The figure shows three views and two pictorial views of one solid part (mm, origin at its lowest corner). Answer the questions. A direction names the side the tool comes from. Coordinates: 2 decimals unless noted, no trailing zeros. Order: outer loops, then holes, each group sorted by start corner. A loop starts at its lowest first (then second) coordinate and runs counter-clockwise, first axis right, second up. Notation, with made-up numbers: M -35.5,74.5 L -4.5,74.5 A31 cw -4.5,109.5 Z; hole C -21,78 d3. An arc over 180 degrees is marked long. Answer in a Markdown table with one row per item. Add a question column.
Item 1: The part is cut by section C-C (y = 11.25). Write down the section's boundary in (x, z).
Item 2: Flat-ended cylindrical pins translate along their axes: pin 1 Ø7.5 at (x, y) = (31, 4.5) entering from -Z; pin 2 Ø4.5 at (y, z) = (6, 13.5) entering from +X. Find the tip coordinate at first contact, or state that the pin passes through.
Item 3: The part is cut by section A-A (x = 4.75). Write down the section's boundary in (y, z).
Item 4: Consider line 1 (Z direction, x = 4.75, y = 7.5); line 2 (Z direction, x = 47.75, y = 10); line 3 (Z direction, x = 22, y = 11.5). Determine where each line is inside the solid, lowest interval first. Write a range as from..to.
Item 5: Which of the six approach directions +Z, -Z, +X, -X, +Y, -Y give full straight-line access (tool end or side, diameter ignored) to the marked faces 1 and 2?
Item 6: The part is cut by section B-B (z = 44.75). Write down the section's boundary in (x, y).
Item 7: The mould has two halves that part along Z. Classify the marked faces 3, 4, 5 and 6: released by +Z, released by -Z, zero draft, split by the parting line, or undercut.
Item 8: The part is cut by section D-D (x = 11). Write down the section's boundary in (y, z).
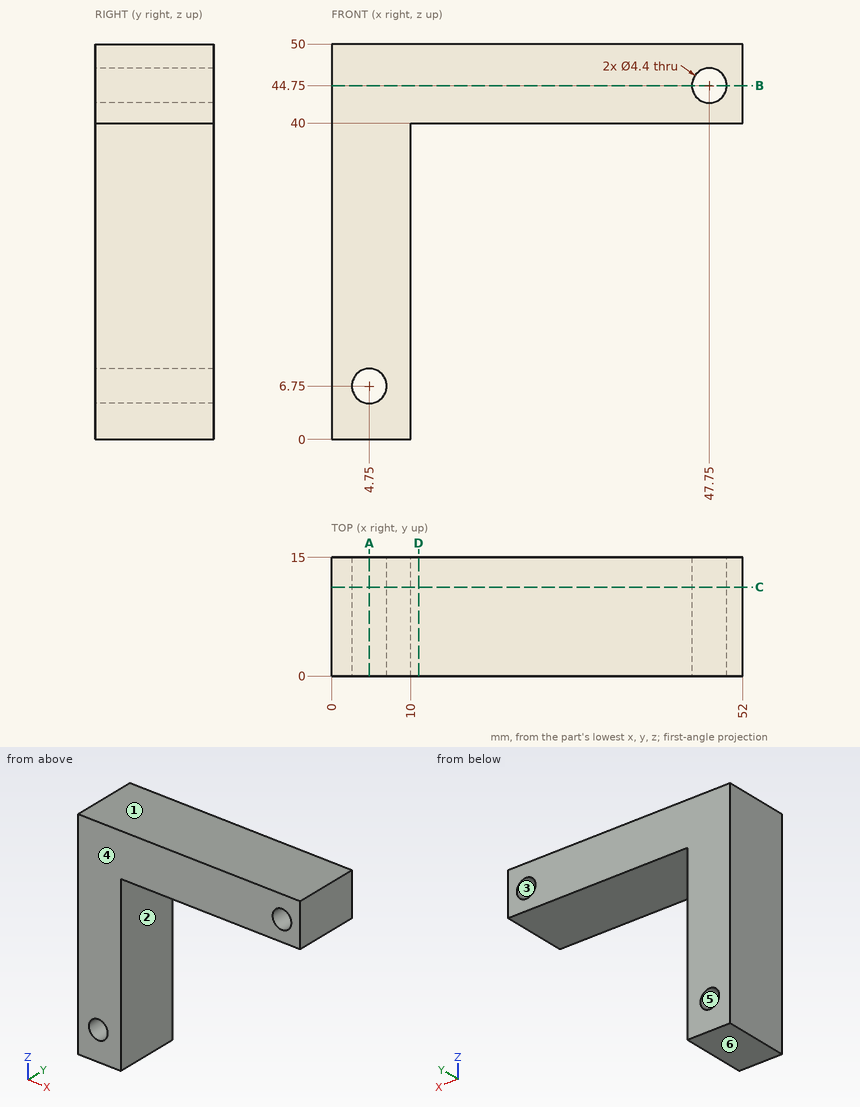
Reply:
| question | item | result |
|---|---|---|
| 1 | outline | M 0,0 L 10,0 L 10,40 L 52,40 L 52,50 L 0,50 Z; hole C 4.75,6.75 d4.4; hole C 47.75,44.75 d4.4 |
| 2 | pin 1 | stops at z = 40 |
| 2 | pin 2 | stops at x = 10 |
| 3 | outline | M 0,0 L 15,0 L 15,4.55 L 0,4.55 Z; M 0,8.95 L 15,8.95 L 15,50 L 0,50 Z |
| 4 | line 1 | z = 0..4.55, 8.95..50 |
| 4 | line 2 | z = 40..42.55, 46.95..50 |
| 4 | line 3 | z = 40..50 |
| 5 | face 1 | +Z, +X, -X, +Y, -Y |
| 5 | face 2 | -Z, +X, +Y, -Y |
| 6 | outline | M 0,0 L 45.55,0 L 45.55,15 L 0,15 Z; M 49.95,0 L 52,0 L 52,15 L 49.95,15 Z |
| 7 | face 3 | undercut |
| 7 | face 4 | zero draft |
| 7 | face 5 | undercut |
| 7 | face 6 | released by -Z |
| 8 | outline | M 0,40 L 15,40 L 15,50 L 0,50 Z |
